Autodesk Inventor part; units mm, degrees
ref_plane "YZ Plane" through (0, 0, 0) normal (1, 0, 0) x (0, 1, 0)
ref_plane "XZ Plane" through (0, 0, 0) normal (0, 1, 0) x (-1, 0, 0)
ref_plane "XY Plane" through (0, 0, 0) normal (0, 0, 1) x (1, 0, 0)
sketch "Sketch1" plane through (0, 0, 0) normal (0, 1, 0) x (-1, 0, 0)
  line L0 (6.5, -2) -> (6.5, -22)
  line L1 (16.25, -22) -> (16.25, -32)
  line L2 (16.25, 0) -> (16.25, -2)
  line L3 (0, 0) -> (0, -32)
  line L4 (16.25, 0) -> (0, 0)
  line L5 (16.25, -2) -> (6.5, -2)
  line L6 (16.25, -22) -> (6.5, -22)
  line L7 (16.25, -32) -> (0, -32)
  point P0 (0, 26.9125)
  point P1 (0, -16.1673)
  point P2 (0, 6.9125)
  point P3 (0, -16)
  dimension "d19" = 20
  dimension "d20" = 10
  dimension "d21" = 2
  dimension "d22" = 32.5
  dimension "d23" = 13
  dimension "d24" = 32.5
revolve "Revolution1" add sketch "Sketch1" angle 360 about axis through (0, 0, 0) along (0, 0, -1)
sketch "Sketch3" plane through (0, 0, -2) normal (0, 0, -1) x (-1, 0, 0)
  circle A0 centre (0, 0) radius 11 construction
  point P0 (0, -11)
  dimension "d25" = 22
hole "Hole2" at (0, -11, -2) direction (0, 0, 1) diameter 4.1 end through all
pattern_circular "Circular Pattern2" count 3 over 360 about axis through (0, 0, -10) along (0, 0, 1) of "Hole2"
sketch "Sketch4" plane through (0, 0, -32) normal (0, 0, -1) x (-1, 0, 0)
  line L0 (9, 0) -> (-9, 0) construction
  point P0 (0, 0)
  point P1 (0, 0)
  dimension "d36" = 18
hole "Hole3" at (-9, 0, -32) at (9, 0, -32) direction (0, 0, 1) diameter 2.459 depth 10
chamfer "Chamfer1" distance 0.2 angle 45 4 edges at (16.25, 0, -32) (16.25, 0, -22) (16.25, 0, -2) (16.25, 0, 0)
equation "\"d23\" = stockid"
equation "\"d25\" = holesid"
equation "\"holesid\" = 22"
equation "\"stockid\" = 13"
properties part number "HayashiProbeHead" material "Stainless Steel"
Input: part model. Units: mm. Frame: model coordinates. A direction names the side the tool comes from. Give positions to 0.01 mm unless a question says otherwise; leave off trailing zeros. Write each loop counter-clockwise with the first axis right and the second up, starting at its lowest first coordinate (ties: lowest second). Pieces come first, ordered by that corner, then holes. Notation, with made-up numbers: (78, 67) - (129, 67) arc R25 cw to (129, 91) - close; hole circle Ø2 at (54.5, 5). An arc over 180 degrees is marked (long way). Write item = value, one per line. Start each with the question number.
1) Pin query (flat end, axial travel): pin 1 (4 mm diameter, centred on x = -7.5, z = -10.5, fed in from -Y); pin 2 (2 mm diameter, centred on x = -8.5, z = -10.5, fed in from +Y); pin 3 (2 mm diameter, centred on x = 9, y = 0, fed in from -Z); pin 4 (4 mm diameter, centred on y = 6.5, z = -11.5, fed in from +X). Return the tip coordinate at first contact, or that it passes through.
2) Cut plane B-B (y = 0). Return loops of the section in (x, z), and give its area (3 significant figures).
3) Cut plane C-C (z = -21.5). Return loops of the section in (x, y), and give its area (3 significant figures).
4) Material intervals for L1, parallel to Z at x = 2, y = -7; L2, parallel to Y at x = 0, z = -0.9; L3, parallel to X at y = 0.5, z = -30, sorted ascending. Write a range as [from, to].
5) Cut plane A-A (x = 0). Return loops of the section in (y, z), and give its area (3 significant figures).
6) Draft query along Z for faces 5 (the face through (0, 0, -32)), 6 (the face through (-7.525, 5.056, -0.986)), 7 (the face through (5.158, -3.955, -12.14)), 8 (the face through (0, -7, -2)). Return one class per face: pulls with the +Z half, pulls with the -Z half, needs draft (parallel to the pull), parting line crosses it, or undercut.
7) Reachability of faces 1 (the face through (0, 0, 0)), 2 (the face through (10.2, -0.27, -26.93)), 3 (the face through (-0.09, -13.05, -0.99)), 4 (the face through (-7, 0, -22)) from +Z, -Z, +X, -X, +Y, -Y: full face, straight path, thin tool, end or side. Return the list, or none.
8) Cut plane D-D (x = -9). Give the number of separate pieces and of enclosed holes in the cut face, and give its area (3 significant figures).
Answers follow:
q1.pin_1 = -3.46
q1.pin_2 = through
q1.pin_3 = -2
q1.pin_4 = 4.69
q2.outline = (-16.25, -31.8) - (-16.05, -32) - (-10.23, -32) - (-10.23, -22) - (-16.05, -22) - (-16.25, -22.2) - close; (-16.25, -1.8) - (-16.05, -2) - (-6.5, -2) - (-6.5, -22) - (-7.77, -22) - (-7.77, -32) - (7.77, -32) - (7.77, -22) - (6.5, -22) - (6.5, -2) - (16.05, -2) - (16.25, -1.8) - (16.25, -0.2) - (16.05, 0) - (-16.05, 0) - (-16.25, -0.2) - close; (10.23, -32) - (16.05, -32) - (16.25, -31.8) - (16.25, -22.2) - (16.05, -22) - (10.23, -22) - close
q2.area = 601 mm^2
q3.outline = circle Ø13 at (0, 0)
q3.area = 133 mm^2
q4.L1 = [-32, -22], [-2, 0]
q4.L2 = [-16.25, -13.05], [-8.95, 16.25]
q4.L3 = [-16.24, -10.12], [-7.88, 7.88], [10.12, 16.24]
q5.outline = (-16.25, -31.8) - (-16.05, -32) - (16.05, -32) - (16.25, -31.8) - (16.25, -22.2) - (16.05, -22) - (6.5, -22) - (6.5, -2) - (16.05, -2) - (16.25, -1.8) - (16.25, -0.2) - (16.05, 0) - (-8.95, 0) - (-8.95, -2) - (-6.5, -2) - (-6.5, -22) - (-16.05, -22) - (-16.25, -22.2) - close; (-16.25, -1.8) - (-16.05, -2) - (-13.05, -2) - (-13.05, 0) - (-16.05, 0) - (-16.25, -0.2) - close
q5.area = 642 mm^2
q6.face_5 = pulls with the -Z half
q6.face_6 = needs draft
q6.face_7 = undercut
q6.face_8 = undercut
q7.face_1 = +Z, +X, -X, +Y, -Y
q7.face_2 = -Z
q7.face_3 = +Z
q7.face_4 = none
q8.separate_pieces = 4
q8.enclosed_holes = 0
q8.area = 292 mm^2
